```python
from build123d import *

# Parameters (mm, degrees)
SKETCH1_W           = 100
SKETCH1_H           = 100
BOSS_EXTRUDE1_DEPTH = 40
SKETCH2_W           = 90
SKETCH2_H           = 90
CUT_EXTRUDE1_DEPTH  = 35
FILLET1_R           = 10


with BuildPart() as part:
    # Sketch1 → Boss-Extrude1 (new body)
    with BuildSketch(Plane(origin=(0, 0, 0), x_dir=(1, 0, 0), z_dir=(0, 1, 0))):
        with Locations((50, -50)):
            Rectangle(SKETCH1_W, SKETCH1_H)
    extrude(amount=BOSS_EXTRUDE1_DEPTH)

    # Sketch2 → Cut-Extrude1 (cut)
    with BuildSketch(Plane(origin=(0, 40, 0), x_dir=(1, 0, 0), z_dir=(0, 1, 0))):
        with Locations((50, -50)):
            Rectangle(SKETCH2_W, SKETCH2_H)
    extrude(amount=-CUT_EXTRUDE1_DEPTH, mode=Mode.SUBTRACT)

    # Fillet1
    fillet1_edges = [part.edges().sort_by_distance(p)[0] for p in [
        (5, 22.5, 95),
        (5, 22.5, 5),
        (95, 22.5, 5),
        (95, 22.5, 95),
        (0, 20, 0),
        (100, 20, 0),
        (100, 20, 100),
        (0, 20, 100),
    ]]
    fillet(fillet1_edges, radius=FILLET1_R)


solid = part.part
```
CAD build for the part. Positions are in the model's coordinates, mm. A direction names the side the tool comes from. Round coordinates to 2 decimals unless told otherwise and drop trailing zeros. Order: outer loops, then holes, each group sorted by start corner. A loop starts at its lowest first (then second) coordinate and runs counter-clockwise, first axis right, second up. Notation, with made-up numbers: (-34.5, 1) - (1.5, 1) arc R25 ccw to (1.5, 39) - close; hole circle Ø10 at (54, -38). An arc over 180 degrees is marked (long way). Use CSV: the item, a comma, the result in double quotes. Start each with the question number.
1) Two-plate mould, pull along X, no slides. Class faces 3 (the cylindrical face through (2.85, 20.28, 96.99)), 4 (the cylindrical face through (96.99, 20.28, 97.15)), 5 (the flat face through (49, 5, 49)), 6 (the flat face through (49, 20, 100)): pulls with the +X half, pulls with the -X half, needs draft (parallel to the pull), parting line crosses it, or undercut.
2) Saw through at B-B (x = 63.5). List the corners of the cut face in (y, z).
3) Wall check: L1, parallel to Z at x = 75.5, y = 19.5; L2, parallel to Y at x = 34, z = 39.5. Give the ranges that are in metal, low to high. Write a range as [from, to].
4) Saw through at C-C (z = 45.5). List the corners of the cut face in (x, y), and give its area (3 significant figures).
5) Tool access for faces 1 (the cylindrical face through (91.99, 22.26, 92.15)), 2 (the cylindrical face through (96.99, 20.28, 2.85)): list every direction of +Z, -Z, +X, -X, +Y, -Y with a clear straight run to the whole face (end or side of a thin tool).
6) Saw through at A-A (y = 26.5). List the corners of the cut face in (x, z).
7) Pin check, flat tip, straight feed: pin 1 Ø6 at (x, z) = (62, 85.5) entering from -Y. Stop position of the tip, or through.
Values follow:
1,face 3,"pulls with the -X half"
1,face 4,"pulls with the +X half"
1,face 5,"undercut"
1,face 6,"needs draft"
2,outline,"(0, 0) - (40, 0) - (40, 5) - (5, 5) - (5, 95) - (40, 95) - (40, 100) - (0, 100) - close"
3,L1,"z = [0, 5], [95, 100]"
3,L2,"y = [0, 5]"
4,outline,"(0, 0) - (100, 0) - (100, 40) - (95, 40) - (95, 5) - (5, 5) - (5, 40) - (0, 40) - close"
4,area,"850 mm2"
5,face 1,"+Y"
5,face 2,"-Z, +X, +Y, -Y"
6,outline,"(0, 10) arc R10 ccw to (10, 0) - (90, 0) arc R10 ccw to (100, 10) - (100, 90) arc R10 ccw to (90, 100) - (10, 100) arc R10 ccw to (0, 90) - close; hole (5, 15) arc R10 ccw to (15, 5) - (85, 5) arc R10 ccw to (95, 15) - (95, 85) arc R10 ccw to (85, 95) - (15, 95) arc R10 ccw to (5, 85) - close"
7,pin 1,"stops at y = 0"
